For this review, take the finished solid that the model builds, in its own axes (mm). A direction names the side the tool comes from. Coordinates: 2 decimals unless noted, no trailing zeros. Loops run counter-clockwise (first coordinate to the right, second up) from the corner with the lowest first, then second, coordinate; pieces in that order, holes last.
```python
from build123d import *

# Parameters (mm, degrees)
F0_W     = 95.25
F0_H     = 75.367778
F0_R     = 23.749
F1_DEPTH = 25.4
F2_R     = 3.5687
F3_DEPTH = 7.1374


with BuildPart() as f1:
    # F0 (on Front) → F1 (new body)
    with BuildSketch(Plane.XZ):
        with Locations((18.133259, -13.926655)):
            Rectangle(F0_W, F0_H)
        with Locations((18.133259, -13.926655)):
            Circle(F0_R, mode=Mode.SUBTRACT)
    extrude(amount=-F1_DEPTH)

    # F2 (on face) → F3 (cut)
    with BuildSketch(Plane.XY.offset(23.757234)):
        with Locations((-23.535441, 12.7)):
            Circle(F2_R)
        with Locations((56.233259, 12.7)):
            Circle(F2_R)
    extrude(amount=-F3_DEPTH, mode=Mode.SUBTRACT)


solid = f1.part
```
Q1. Consider section B-B (y = 13.75). State the section outline as (x, z) points, then the cut area to 3 significant figures.
Q2. Consider section C-C (x = 10.5). State the section outline as (y, z) points.
Q3. The part is to be moulded in two halves that separate along Y. For faces 1 (the face through (-29.492, 13, -14)), 2 (the face through (17, 25.4, 12)), 3 (the face through (56, 13, 16.62)), say which applies: +Y half, -Y half, draft (parallel to the pull), parting line (faces both ways), or undercut.
Q4. For pin 1 Ø11.5 at (x, y) = (56.23, 12.7) entering from +Z, flat-tipped, find the tip position at first contact; note if it passes through.
Q5. Machinability: for faces 4 (the face through (-26.37, 10.53, 20.24)), 5 (the face through (17, 13, -51.611)), which of the approach directions +Z, -Z, +X, -X, +Y, -Y give a long, thin tool a straight path to every point of the face, cutting with its end or side? Answer none if there is none.
Q6. Consider section A-A (z = 2). State the section outline as (x, y) points, then the cut area to 3 significant figures.
Q7. Wall thickness on probe 1 along Z at (x, y) = (18.5, 24.25); probe 2 along Z at (x, y) = (4.5, 4.5); probe 3 along X at (y, z) = (3, -11): over which ranges is each line inside the solid? List them lowest first.
Q8. Consider section D-D (y = 2). State the section outline as (x, z) points.
Model answer:
1. outline: (-29.49, -51.61) - (65.76, -51.61) - (65.76, 23.76) - (59.64, 23.76) - (59.64, 16.62) - (52.82, 16.62) - (52.82, 23.76) - (-20.12, 23.76) - (-20.12, 16.62) - (-26.95, 16.62) - (-26.95, 23.76) - (-29.49, 23.76) - close; hole circle Ø47.5 at (18.13, -13.93)
1. area: 5,310 mm2
2. outline: (0, -51.61) - (25.4, -51.61) - (25.4, -36.42) - (0, -36.42) - close; (0, 8.56) - (25.4, 8.56) - (25.4, 23.76) - (0, 23.76) - close
3. face 1: draft
3. face 2: +Y half
3. face 3: undercut
4. pin 1: stops at z = 23.76
5. face 4: +Z
5. face 5: -Z, +X, -X, +Y, -Y
6. outline: (-29.49, 0) - (0.52, 0) - (0.52, 25.4) - (-29.49, 25.4) - close; (35.75, 0) - (65.76, 0) - (65.76, 25.4) - (35.75, 25.4) - close
6. area: 1,520 mm2
7. probe 1: z = -51.61 to -37.67, 9.82 to 23.76
7. probe 2: z = -51.61 to -33.37, 5.52 to 23.76
7. probe 3: x = -29.49 to -5.43, 41.7 to 65.76
8. outline: (-29.49, -51.61) - (65.76, -51.61) - (65.76, 23.76) - (-29.49, 23.76) - close; hole circle Ø47.5 at (18.13, -13.93)
